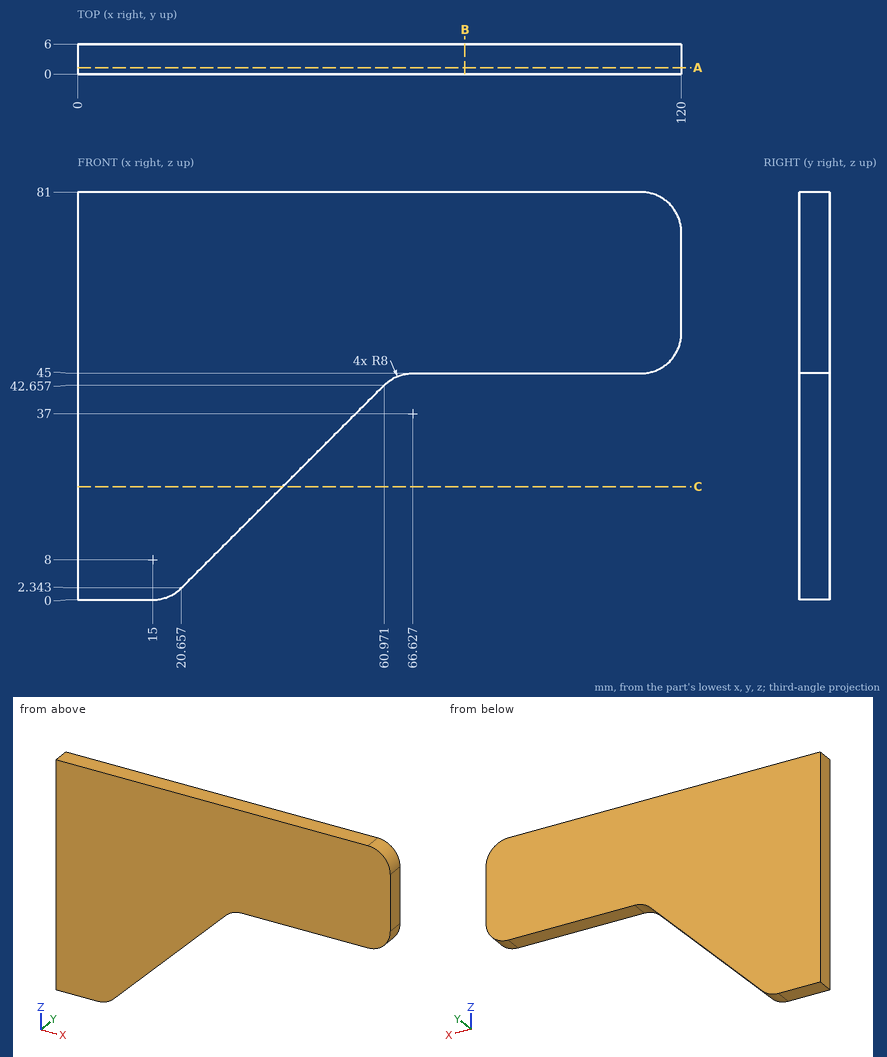
Can you work these out from the drawing? Everything is in mm from the part's minimum corner. Give positions to 0.01 mm unless a question says otherwise; leave off trailing zeros. Loops run counter-clockwise (first coordinate to the right, second up) from the corner with the lowest first, then second, coordinate; pieces in that order, holes last. Notation, with made-up numbers: (60, -31.5) -> (89, -31.5) arc R33 ccw to (89, 2.5) -> close; hole circle Ø2 at (88, -38). An arc over 180 degrees is marked (long way). Return JSON: item names as keys, results as strings.
Item 1: If we section it at B-B on x = 77: List the corners of the cut face in (y, z) for me.
Geometry results:
{"outline": "(0, 45) -> (6, 45) -> (6, 81) -> (0, 81) -> close"}
Item 2: I need wall thicknesses on L1, parallel to Z at x = 95, y = 2.15; L2, parallel to X at y = 0.9, z = 15 (1 decimal); L3, parallel to X at y = 4.3, z = 30 (1 decimal). Which ranges of each line are inside material? Lowest first, please. Write a range as from..to.
Geometry results:
{"L1": "z = 45..81", "L2": "x = 0..33.3", "L3": "x = 0..48.3"}
Item 3: I'm going to push flat-ended pins straight in: pin 1 (1.5 mm diameter, centred on y = 3, z = 10.5, fed in from +X) (1 decimal); pin 2 (2 mm diameter, centred on x = 67, y = 3, fed in from -Z) (1 decimal). Where does each tip first touch, or does it pass through?
Geometry results:
{"pin 1": "stops at x = 29.6", "pin 2": "stops at z = 45"}
Item 4: If we section it at C-C on z = 22.5: List the corners of the cut face in (x, y) for me.
Geometry results:
{"outline": "(0, 0) -> (40.81, 0) -> (40.81, 6) -> (0, 6) -> close"}
Item 5: If we section it at A-A on y = 1.3: List the corners of the cut face in (x, z) for me.
Geometry results:
{"outline": "(0, 0) -> (15, 0) arc R8 ccw to (20.66, 2.34) -> (60.97, 42.66) arc R8 cw to (66.63, 45) -> (112, 45) arc R8 ccw to (120, 53) -> (120, 73) arc R8 ccw to (112, 81) -> (0, 81) -> close"}
